Build history of the part. All positions in model axes, mm. A direction names the side the tool comes from. Round coordinates to 2 decimals unless told otherwise and drop trailing zeros. Loops run counter-clockwise (first coordinate to the right, second up) from the corner with the lowest first, then second, coordinate; pieces in that order, holes last. Notation, with made-up numbers: M -12,18.5 L -1,18.5 A29 cw -1,43.5 Z; hole C 76.5,69 d1. An arc over 180 degrees is marked long. One line per item, written item: value.
```python
from build123d import *

# Parameters (mm, degrees)
SKETCH1_W           = 171.45
SKETCH1_H           = 101.6
BOSS_EXTRUDE1_DEPTH = 21.59
SKETCH2_W           = 158.75
SKETCH2_H           = 90.424
CUT_EXTRUDE1_DEPTH  = 11.43
FILLET1_R           = 5.08
FILLET2_R           = 10.16


with BuildPart() as part:
    # Sketch1 → Boss-Extrude1 (new body)
    with BuildSketch(Plane(origin=(0, 0, 0), x_dir=(1, 0, 0), z_dir=(0, 1, 0))):
        Rectangle(SKETCH1_W, SKETCH1_H)
    extrude(amount=BOSS_EXTRUDE1_DEPTH)

    # Sketch2 → Cut-Extrude1 (cut)
    with BuildSketch(Plane(origin=(0, 21.59, 0), x_dir=(1, 0, 0), z_dir=(0, 1, 0))):
        Rectangle(SKETCH2_W, SKETCH2_H)
    extrude(amount=-CUT_EXTRUDE1_DEPTH, mode=Mode.SUBTRACT)

    # Fillet1
    fillet1_edges = [part.edges().sort_by_distance(p)[0] for p in [
        (-79.375, 15.875, 45.212),
        (-79.375, 15.875, -45.212),
        (79.375, 15.875, -45.212),
        (79.375, 15.875, 45.212),
    ]]
    fillet(fillet1_edges, radius=FILLET1_R)

    # Fillet2
    fillet2_edges = [part.edges().sort_by_distance(p)[0] for p in [
        (-85.725, 10.795, -50.8),
        (85.725, 10.795, -50.8),
        (85.725, 10.795, 50.8),
        (-85.725, 10.795, 50.8),
    ]]
    fillet(fillet2_edges, radius=FILLET2_R)


solid = part.part
```
Item 1: Pull direction X, two halves, no side cores. Call faces 3 (the face through (-1, 16, -45.212)), 4 (the face through (85.725, 11, 1)), 5 (the face through (-77.85, 15.79, -43.76)), 6 (the face through (-85.725, 11, 1)): pulls with the +X half, pulls with the -X half, needs draft (parallel to the pull), parting line crosses it, or undercut.
Check values:
face 3: undercut
face 4: pulls with the +X half
face 5: undercut
face 6: pulls with the -X half
Item 2: Wall check: line 1 along Z through (x, y) = (73, 12.75); line 2 along X through (y, z) = (11, -27) (3 decimals); line 3 along Y through (x, z) = (-47.5, -32). Give the ranges that are in metal, low to high.
Check values:
line 1: z = -50.8 to -45.21, 45.21 to 50.8
line 2: x = -85.725 to -79.375, 79.375 to 85.725
line 3: y = 0 to 10.16
Item 3: Slice it at C-C, the plane z = 24.5. Give the cut face in (x, y) (3 decimals).
Check values:
outline: M -85.725,0 L 85.725,0 L 85.725,21.59 L 79.375,21.59 L 79.375,10.16 L -79.375,10.16 L -79.375,21.59 L -85.725,21.59 Z
Item 4: Drop a flat-ended pin along its axis: P1, Ø8, axis at x = 35.5, z = 12.5, coming from the +Y side. Give the stop position or say it passes through.
Check values:
P1: stops at y = 10.16
Item 5: Slice it at B-B, the plane x = 47. Give the cut face in (y, z).
Check values:
outline: M 0,-50.8 L 21.59,-50.8 L 21.59,-45.21 L 10.16,-45.21 L 10.16,45.21 L 21.59,45.21 L 21.59,50.8 L 0,50.8 Z
Item 6: Which spindle directions (+Z, -Z, +X, -X, +Y, -Y) get a long thin tool onto all of the face, cutting with end or side? Do faces 1 (the face through (-1, 11, -50.8)), 2 (the face through (79.375, 16, 1)). Say none if no direction does.
Check values:
face 1: -Z, +X, -X, +Y, -Y
face 2: +Y
Item 7: Slice it at A-A, the plane y = 12. Give the cut face in (x, z) (3 decimals), and give its area (3 significant figures).
Check values:
outline: M -85.725,-40.64 A10.16 ccw -75.565,-50.8 L 75.565,-50.8 A10.16 ccw 85.725,-40.64 L 85.725,40.64 A10.16 ccw 75.565,50.8 L -75.565,50.8 A10.16 ccw -85.725,40.64 Z; hole M -79.375,-40.132 A5.08 ccw -74.295,-45.212 L 74.295,-45.212 A5.08 ccw 79.375,-40.132 L 79.375,40.132 A5.08 ccw 74.295,45.212 L -74.295,45.212 A5.08 ccw -79.375,40.132 Z
area: 3,000 mm2
